Build history of the part. All positions in model axes, mm. A direction names the side the tool comes from. Round coordinates to 2 decimals unless told otherwise and drop trailing zeros. Write each loop counter-clockwise with the first axis right and the second up, starting at its lowest first coordinate (ties: lowest second). Pieces come first, ordered by that corner, then holes. Notation, with made-up numbers: M -4.5,-3 L 37.5,-3 A16 cw 37.5,4 Z; hole C 62,-15.75 d1. An arc over 180 degrees is marked long. Use a Markdown table: item, result.
from build123d import *

# Parameters (mm, degrees)
F1_DEPTH = 23.8125
F3_DEPTH = 25.4
F5_DEPTH = 25.4


with BuildPart() as f1:
    # F0 (on Right) → F1 (new body)
    with BuildSketch(Plane.YZ):
        Polygon((30.8235474857, 22.3946181123), (0, 0), (-38.1, 0), (-38.1, -3.175), (1.0316200355, -3.175), (32.6897656617, 19.8259891552), align=None)
    extrude(amount=F1_DEPTH)

    # F2 (on face) → F3 (cut)
    with BuildSketch(Plane.XY):
        with BuildLine():
            ThreePointArc((11.90625, -23.01875), (9.525, -25.4), (11.90625, -27.78125))
            Line((11.90625, -27.78125), (11.90625, -23.01875))
        make_face()
        with BuildLine():
            ThreePointArc((11.90625, -10.31875), (9.525, -12.7), (11.90625, -15.08125))
            Line((11.90625, -15.08125), (11.90625, -10.31875))
        make_face()
        with BuildLine():
            Line((11.90625, -10.31875), (11.90625, -15.08125))
            ThreePointArc((11.90625, -15.08125), (13.5900480227, -14.3837980227), (14.2875, -12.7))
            ThreePointArc((14.2875, -12.7), (13.5900480227, -11.0162019773), (11.90625, -10.31875))
        make_face()
        with BuildLine():
            Line((11.90625, -23.01875), (11.90625, -27.78125))
            ThreePointArc((11.90625, -27.78125), (13.5900480227, -27.0837980227), (14.2875, -25.4))
            ThreePointArc((14.2875, -25.4), (13.5900480227, -23.7162019773), (11.90625, -23.01875))
        make_face()
    extrude(amount=-F3_DEPTH, mode=Mode.SUBTRACT)

    # F4 (on face) → F5 (cut)
    with BuildSketch(Plane(origin=(0, 0, 0), x_dir=(1, 0, 0), z_dir=(0, -0.5877852523, 0.8090169944))):
        with BuildLine():
            ThreePointArc((11.90625, 15.08125), (9.525, 12.7), (11.90625, 10.31875))
            Line((11.90625, 10.31875), (11.90625, 15.08125))
        make_face()
        with BuildLine():
            ThreePointArc((11.90625, 27.78125), (9.525, 25.4), (11.90625, 23.01875))
            Line((11.90625, 23.01875), (11.90625, 27.78125))
        make_face()
        with BuildLine():
            Line((11.90625, 27.78125), (11.90625, 23.01875))
            ThreePointArc((11.90625, 23.01875), (13.5900480227, 23.7162019773), (14.2875, 25.4))
            ThreePointArc((14.2875, 25.4), (13.5900480227, 27.0837980227), (11.90625, 27.78125))
        make_face()
        with BuildLine():
            Line((11.90625, 15.08125), (11.90625, 10.31875))
            ThreePointArc((11.90625, 10.31875), (13.5900480227, 11.0162019773), (14.2875, 12.7))
            ThreePointArc((14.2875, 12.7), (13.5900480227, 14.3837980227), (11.90625, 15.08125))
        make_face()
    extrude(amount=-F5_DEPTH, mode=Mode.SUBTRACT)


solid = f1.part
Q1. Cut at D-D on x = 10.25. Give the cut face in (y, z) (3 decimals), and give its area (3 significant figures).
Response values:
| item | result |
|---|---|
| outline | M -38.1,-3.175 L -27.111,-3.175 L -27.111,0 L -38.1,0 Z; M -23.689,-3.175 L -14.411,-3.175 L -14.411,0 L -23.689,0 Z; M -10.989,-3.175 L 1.032,-3.175 L 10.757,3.891 L 8.89,6.459 L 0,0 L -10.989,0 Z; M 11.659,8.471 L 13.525,5.902 L 21.031,11.355 L 19.165,13.924 Z; M 21.933,15.935 L 23.799,13.367 L 32.69,19.826 L 30.824,22.395 Z |
| area | 202 mm2 |
Q2. Drill centre lines: L1, parallel to X at y = -12.7, z = -1.5 (1 decimal); L2, parallel to Z at x = 18.5, y = -0.5 (3 decimals); L3, parallel to Y at x = 18.5, z = 8. Where is each one in solid material? Low to high.
Response values:
| item | result |
|---|---|
| L1 | x = 0 to 9.5, 14.3 to 23.8 |
| L2 | z = -3.175 to 0 |
| L3 | y = 11.01 to 16.41 |
Q3. Which spindle directions (+Z, -Z, +X, -X, +Y, -Y) get a long thin tool onto all of the face, cutting with end or side? Do faces 1 (the flat face through (12, -19, 0)), 2 (the cylindrical face through (10.15, 22.77, 14.61)). Say none if no direction does.
Response values:
| item | result |
|---|---|
| face 1 | +Z, +X, -X, -Y |
| face 2 | none |
Q4. Drop flat-ended pins along their axis: P1, Ø8, axis at x = 14.5, z = -0.5, coming from the +Y side; P2, Ø10, axis at x = 7, y = -6, coming from the +Z side; P3, Ø1.5, axis at x = 15, y = 9.5, coming from the +Z side. Give the stop position or say it passes through.
Response values:
| item | result |
|---|---|
| P1 | stops at y = 10.22 |
| P2 | stops at z = 0 |
| P3 | stops at z = 7.45 |
Q5. Two-plate mould, pull along X, no slides. Class faces 3 (the cylindrical face through (13.01, -14.81, -1.57)), 4 (the flat face through (0, 2, 1)), 5 (the flat face through (12, -38.1, -2)): +X half, -X half, draft (parallel to the pull), parting line (faces both ways), or undercut.
Response values:
| item | result |
|---|---|
| face 3 | undercut |
| face 4 | -X half |
| face 5 | draft |
Q6. Cut at C-C on z = -1. Give the cut face in (x, y).
Response values:
| item | result |
|---|---|
| outline | M 0,-38.1 L 23.81,-38.1 L 23.81,4.03 L 0,4.03 Z; hole C 11.91,-25.4 d4.76; hole C 11.91,-12.7 d4.76 |
Q7. Cut at A-A on y = -12.7. Give the cut face in (x, z) (1 decimal).
Response values:
| item | result |
|---|---|
| outline | M 0,-3.2 L 9.5,-3.2 L 9.5,0 L 0,0 Z; M 14.3,-3.2 L 23.8,-3.2 L 23.8,0 L 14.3,0 Z |
Q8. Cut at B-B on x = 5.5. Give the cut face in (y, z) (3 decimals), and give its area (3 significant figures).
Response values:
| item | result |
|---|---|
| outline | M -38.1,-3.175 L 1.032,-3.175 L 32.69,19.826 L 30.824,22.395 L 0,0 L -38.1,0 Z |
| area | 245 mm2 |
